Input: part model. Units: mm. Frame: model coordinates. Round coordinates to 2 decimals unless told otherwise and drop trailing zeros. Loops run counter-clockwise (first coordinate to the right, second up) from the corner with the lowest first, then second, coordinate; pieces in that order, holes last. Notation, with made-up numbers: (-20.75, 62.25) -> (-4.75, 62.25) arc R32 ccw to (-4.75, 90.25) -> close; hole circle Ø10 at (-23, 82.5). An arc over 180 degrees is marked (long way). Answer as a JSON object with one key per item and string values. Group by question number.
Item 1: Section query A-A on x = 1.5. Count the separate pieces of the cut face and the enclosed holes in it, and give its area (3 significant figures).
Item 2: Material intervals for line 1 (Y direction, x = 7.45, z = -102.5); line 2 (Z direction, x = 8.95, y = -2); line 3 (Y direction, x = 2.25, z = 107.5), sorted ascending. Write a range as [from, to].
Item 3: Pin query (flat end, axial travel): pin 1 (3.5 mm diameter, centred on y = -35, z = 1, fed in from +X); pin 2 (2.5 mm diameter, centred on y = -2, z = -102.5, fed in from +X); pin 3 (2 mm diameter, centred on x = 8.5, y = -25, fed in from -Z). Return the tip coordinate at first contact, or that it passes through.
Item 4: Section query B-B on y = 5.5. Return loops of the section in (x, z).
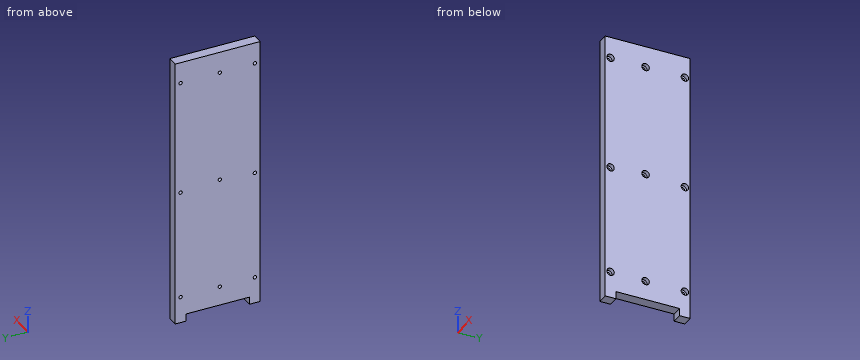
Autodesk Inventor part; units mm, degrees
ref_plane "YZ Plane" through (0, 0, 0) normal (1, 0, 0) x (0, 1, 0)
ref_plane "XZ Plane" through (0, 0, 0) normal (0, 1, 0) x (-1, 0, 0)
ref_plane "XY Plane" through (0, 0, 0) normal (0, 0, 1) x (1, 0, 0)
sketch "Skizze1" plane through (0, 0, 0) normal (1, 0, 0) x (0, 1, 0)
  line L0 (-40, 127.5) -> (40, 127.5)
  line L1 (40, 127.5) -> (40, -127.5)
  line L2 (40, -127.5) -> (-40, -127.5)
  line L3 (-40, -127.5) -> (-40, 127.5)
  line L4 (-40, 127.5) -> (40, -127.5) construction
  line L5 (40, 127.5) -> (-40, -127.5) construction
  point P0 (0, 0)
  dimension "d0" = 80
  dimension "d1" = 255
extrude "Extrusion1" add sketch "Skizze1" along normal blind 10
sketch "Skizze2" plane through (10, 0, 0) normal (1, 0, 0) x (0, 0, -1)
  line L0 (-127.5, 40) -> (-127.5, -40)
  line L1 (127.5, -40) -> (127.5, 40)
  line L2 (127.5, 40) -> (-127.5, 40)
  line L3 (-127.5, -35) -> (127.5, -35) construction
  line L4 (-127.5, -40) -> (127.5, -40)
  line L5 (178.5, 0) -> (-178.5, 0)
  point P0 (0, 0)
  point P1 (-107.5, -2)
  point P2 (-2.5, -2)
  point P3 (102.5, -2)
  point P4 (-107.5, -35)
  point P5 (0, -35)
  point P6 (102.5, -35)
  point P7 (-107.5, 35)
  point P8 (0, 35)
  point P9 (102.5, 35)
  dimension "d4" = 20
  dimension "d5" = 25
  dimension "d6" = 105
  dimension "d7" = 42
  dimension "d8" = 42
  dimension "d9" = 42
  dimension "d27" = 5
hole "Bohrung1" at (10, -2, 107.5) at (10, -2, 2.5) at (10, -2, -102.5) at (10, -35, 107.5) at (10, -35, 0) at (10, -35, -102.5) at (10, 35, -102.5) at (10, 35, 0) at (10, 35, 107.5) direction (-1, 0, 0) diameter 3.242 end through all counterbore diameter 7 counterbore depth 4
sketch "Skizze5" plane through (10, 0, 0) normal (1, 0, 0) x (0, 0, -1)
  line L0 (127.5, -40) -> (127.5, 40)
  line L1 (127.5, -30) -> (120.5, -30)
  line L2 (120.5, -30) -> (120.5, 30)
  line L3 (120.5, 30) -> (127.5, 30)
  line L4 (127.5, 30) -> (127.5, -30)
  line L5 (-127.5, -40) -> (127.5, -40)
  point P0 (0, 0)
  point P1 (124, -30)
  point P2 (124, 30)
  dimension "d28" = 7
  dimension "d29" = 60
  dimension "d30" = 10
extrude "Extrusion2" cut sketch "Skizze5" against normal blind 10
properties part number "ER_Wand_1"
Solved:
{
 "1": {"separate pieces": "1", "enclosed holes": "9", "area": "19,900 mm²"},
 "2": {"line 1": "[-40, -38.5], [-31.5, -5.5], [1.5, 31.5], [38.5, 40]", "line 2": "[-120.5, -106], [-99, -1], [6, 104], [111, 127.5]", "line 3": "[-40, -36.62], [-33.38, -3.62], [-0.38, 33.38], [36.62, 40]"},
 "3": {"pin 1": "x = 6", "pin 2": "through", "pin 3": "z = -120.5"},
 "4": {"outline": "(0, -120.5) -> (10, -120.5) -> (10, 127.5) -> (0, 127.5) -> close"}
}
